Geometry check sheet. Reference: the model listing, model coordinates, mm. Round coordinates to 2 decimals unless told otherwise and drop trailing zeros. Write each loop counter-clockwise with the first axis right and the second up, starting at its lowest first coordinate (ties: lowest second). Pieces come first, ordered by that corner, then holes. Notation, with made-up numbers: M 67.5,66 L 74.5,66 A20 ccw 74.5,83 Z; hole C 81,49.5 d8. An arc over 180 degrees is marked long. One line per item, written item: value. Start each with the question number.
1. Release check for a two-part mould opening along Z. For faces 1 (the flat face through (5, 20, -15)), 2 (the cylindrical face through (3, 2, -1)), 3 (the cylindrical face through (2.46, 37.08, -5.86)), 4 (the cylindrical face through (2.465, 36.038, -26.996)) record: pulls with the +Z half, pulls with the -Z half, needs draft (parallel to the pull), parting line crosses it, or undercut.
2. Section check A-A (x = 3.55). Record the boundary of the cut face in (y, z), and give its area (3 significant figures).
3. Section check B-B (z = -25.5). Record the boundary of the cut face in (x, y).
4. Scan lines: probe 1 along Z at (x, y) = (3.6, 5); probe 2 along Z at (x, y) = (4.15, 4); probe 3 along Y at (x, z) = (1.8, -6.5). Record each from-to range of solid material in increasing order. Write a range as [from, to].
5. Depth check by flat-ended pin: P1, Ø3.5, axis at y = 5, z = -5, coming from the -X side; P2, Ø5, axis at y = 35, z = -25, coming from the +X side. Enter the tip coordinate at first touch or a pass-through.
from build123d import *

# Parameters (mm, degrees)
SKETCH_1_W                 = 30
SKETCH_1_H                 = 40
EXTRUDE_1_DEPTH            = 5
HOLE_WIZARD_M4_1_OUTLINE_R = 2.25
HOLE_WIZARD_M4_1_DEPTH     = 5
FILLET_1_R                 = 5


# Read off the part's stored shape, not the designer's step: M4 间隙孔1
with BuildPart() as part:
    # 草图1 → 凸台-拉伸1 (new body)
    with BuildSketch(Plane(origin=(0, 0, 0), x_dir=(0, 0, -1), z_dir=(1, 0, 0))):
        with Locations((15, 20)):
            Rectangle(SKETCH_1_W, SKETCH_1_H)
    extrude(amount=EXTRUDE_1_DEPTH)

    # M4 间隙孔1 outline → M4 间隙孔1 (cut)
    with BuildSketch(Plane.YZ):
        with Locations((35, -5)):
            Circle(HOLE_WIZARD_M4_1_OUTLINE_R)
        with Locations((5, -25)):
            Circle(HOLE_WIZARD_M4_1_OUTLINE_R)
        with Locations((5, -5)):
            Circle(HOLE_WIZARD_M4_1_OUTLINE_R)
        with Locations((35, -25)):
            Circle(HOLE_WIZARD_M4_1_OUTLINE_R)
    extrude(amount=HOLE_WIZARD_M4_1_DEPTH, mode=Mode.SUBTRACT)

    # 圆角1
    fillet_1_edges = [part.edges().sort_by_distance(p)[0] for p in [
        (2.5, 40, 0),
        (2.5, 40, -30),
        (2.5, 0, -30),
        (2.5, 0, 0),
    ]]
    fillet(fillet_1_edges, radius=FILLET_1_R)


solid = part.part
Result sheet:
1. face 1: needs draft
1. face 2: pulls with the +Z half
1. face 3: undercut
1. face 4: undercut
2. outline: M 0,-25 A5 ccw 5,-30 L 35,-30 A5 ccw 40,-25 L 40,-5 A5 ccw 35,0 L 5,0 A5 ccw 0,-5 Z; hole C 5,-25 d4.5; hole C 5,-5 d4.5; hole C 35,-25 d4.5; hole C 35,-5 d4.5
2. area: 1,110 mm2
3. outline: M 0,0.03 L 5,0.03 L 5,2.81 L 0,2.81 Z; M 0,7.19 L 5,7.19 L 5,32.81 L 0,32.81 Z; M 0,37.19 L 5,37.19 L 5,39.97 L 0,39.97 Z
4. probe 1: z = [-30, -27.25], [-22.75, -7.25], [-2.75, 0]
4. probe 2: z = [-29.9, -27.02], [-22.98, -7.02], [-2.98, -0.1]
4. probe 3: y = [0, 3.32], [6.68, 33.32], [36.68, 40]
5. P1: passes through
5. P2: stops at x = 5
